Verification items for the finished model (mm, model axes). A direction names the side the tool comes from. Give positions to 0.01 mm unless a question says otherwise; leave off trailing zeros. Loops run counter-clockwise (first coordinate to the right, second up) from the corner with the lowest first, then second, coordinate; pieces in that order, holes last. Notation, with made-up numbers: (53.25, 12.25) - (62.25, 12.25) arc R14 cw to (62.25, 28.25) - close; hole circle Ø4 at (71.5, -23.75). An arc over 180 degrees is marked (long way). Put each result on its own line as item: value. Start each with the question number.
```python
from build123d import *

# Parameters (mm, degrees)
SKETCH_2_R          = 1
CUT_EXTRUDE_1_DEPTH = 5


with BuildPart() as part:
    # 草图1 → 旋转1 (revolve)
    with BuildSketch(Plane.XY):
        Polygon((-15.499429975, 0), (21.500570025, 0), (21.500570025, 4), (6.500570025, 4), (6.500570025, 5), (4.500570025, 5), (4.500570025, 3.95), (-12.499429975, 3.95), (-12.499429975, 3.75), (-13.399429975, 3.75), (-13.399429975, 3.95), (-15.499429975, 3.95), align=None)
    revolve(axis=Axis((-15.499429975, 0, 0), (1, 0, 0)))

    # 草图2 → 切除-拉伸1 (cut, symmetric)
    with BuildSketch(Plane(origin=(0, 0, 0), x_dir=(1, 0, 0), z_dir=(0, 1, 0))):
        with Locations((18.500570025, 0)):
            Circle(SKETCH_2_R)
    extrude(amount=CUT_EXTRUDE_1_DEPTH, both=True, mode=Mode.SUBTRACT)


solid = part.part
```
1) Section check D-D, the plane z = 2. Enter the section's corners in (x, y), plus the area to 3 significant figures.
2) Set-up check for faces 4 (the face through (13.896, 3.695, -1.532)), 5 (the face through (21.501, 0, 0)), 6 (the face through (-4.118, -3.135, -2.404)): record each of +Z, -Z, +X, -X, +Y, -Y from which the full face is reachable in a straight line by a thin tool's end or side.
3) Draft check along X on faces 1 (the face through (4.501, 4, 2)), 2 (the face through (5.49, -1.08, -4.88)), 3 (the face through (-12.956, -3.746, 0.165)). Enter one of: pulls with the +X half, pulls with the -X half, needs draft (parallel to the pull), parting line crosses it, or undercut.
4) Section check B-B, the plane y = 0. Enter the section's corners in (x, z).
5) Depth check by flat-ended pin: P1, Ø6, axis at x = -5.5, y = 3, coming from the -Z side; P2, Ø3, axis at x = 15, z = 4, coming from the -Y side; P3, Ø1.5, axis at x = -0.5, z = 0, coming from the -Y side. Enter the tip coordinate at first touch or a pass-through.
6) Scan lines: line 1 along X through (y, z) = (1, 0); line 2 along Z through (x, y) = (-9.5, 0); line 3 along X through (y, z) = (-2.75, 4). Record each from-to range of solid material in increasing order. Write a range as from..to.
7) Section check A-A, the plane z = 0. Enter the section's corners in (x, y).
8) Section check C-C, the plane x = 16. Enter the section's corners in (y, z).
Results are:
1. outline: (-15.5, -3.41) - (-13.4, -3.41) - (-13.4, -3.17) - (-12.5, -3.17) - (-12.5, -3.41) - (4.5, -3.41) - (4.5, -4.58) - (6.5, -4.58) - (6.5, -3.46) - (21.5, -3.46) - (21.5, 3.46) - (6.5, 3.46) - (6.5, 4.58) - (4.5, 4.58) - (4.5, 3.41) - (-12.5, 3.41) - (-12.5, 3.17) - (-13.4, 3.17) - (-13.4, 3.41) - (-15.5, 3.41) - close
1. area: 258 mm2
2. face 4: +X
2. face 5: +Z, -Z, +X, +Y, -Y
2. face 6: -X
3. face 1: pulls with the -X half
3. face 2: needs draft
3. face 3: undercut
4. outline: (-15.5, -3.95) - (-13.4, -3.95) - (-13.4, -3.75) - (-12.5, -3.75) - (-12.5, -3.95) - (4.5, -3.95) - (4.5, -5) - (6.5, -5) - (6.5, -4) - (21.5, -4) - (21.5, 4) - (6.5, 4) - (6.5, 5) - (4.5, 5) - (4.5, 3.95) - (-12.5, 3.95) - (-12.5, 3.75) - (-13.4, 3.75) - (-13.4, 3.95) - (-15.5, 3.95) - close; hole circle Ø2 at (18.5, 0)
5. P1: stops at z = -3.95
5. P2: stops at y = -3.12
5. P3: stops at y = -3.95
6. line 1: x = -15.5..17.5, 19.5..21.5
6. line 2: z = -3.95..3.95
6. line 3: x = 4.5..6.5
7. outline: (-15.5, -3.95) - (-13.4, -3.95) - (-13.4, -3.75) - (-12.5, -3.75) - (-12.5, -3.95) - (4.5, -3.95) - (4.5, -5) - (6.5, -5) - (6.5, -4) - (17.5, -4) - (17.5, 4) - (6.5, 4) - (6.5, 5) - (4.5, 5) - (4.5, 3.95) - (-12.5, 3.95) - (-12.5, 3.75) - (-13.4, 3.75) - (-13.4, 3.95) - (-15.5, 3.95) - close; (19.5, -4) - (21.5, -4) - (21.5, 4) - (19.5, 4) - close
8. outline: circle Ø8 at (0, 0)
